from build123d import *

# Parameters (mm, degrees)
SKETCH1_W           = 85
SKETCH1_H           = 70
SKETCH1_R           = 1.375
SKETCH1_R_2         = 4.125
SKETCH1_R_3         = 3
SKETCH1_R_4         = 1.875
SKETCH1_R_5         = 2
BOSS_EXTRUDE4_DEPTH = 4
SKETCH1_7_R         = 4.5
CUT_EXTRUDE2_DEPTH  = 2


with BuildPart() as part:
    # Sketch1 → Boss-Extrude4 (new body)
    with BuildSketch(Plane(origin=(0, 0, 0), x_dir=(1, 0, 0), z_dir=(0, 1, 0))):
        Rectangle(SKETCH1_W, SKETCH1_H)
        with Locations((-27.5, 25)):
            Circle(SKETCH1_R, mode=Mode.SUBTRACT)
        with Locations((22.5, 25)):
            Circle(SKETCH1_R, mode=Mode.SUBTRACT)
        with Locations((22.5, -24.60667729)):
            Circle(SKETCH1_R, mode=Mode.SUBTRACT)
        with Locations((-27.5, -24.60667729)):
            Circle(SKETCH1_R, mode=Mode.SUBTRACT)
        with Locations((-15.52, 1)):
            Circle(SKETCH1_R_2, mode=Mode.SUBTRACT)
        with Locations((16.478339488, 0.999882702)):
            Circle(SKETCH1_R_3, mode=Mode.SUBTRACT)
        with Locations((9.407211052, 18.471043068)):
            Circle(SKETCH1_R_4, mode=Mode.SUBTRACT)
        with Locations((9.401398241, -16.528956449)):
            Circle(SKETCH1_R_5, mode=Mode.SUBTRACT)
    extrude(amount=BOSS_EXTRUDE4_DEPTH)

    # Sketch1_7 → Cut-Extrude2 (cut)
    with BuildSketch(Plane(origin=(0, 0, 0), x_dir=(1, 0, 0), z_dir=(0, 1, 0))):
        with Locations((16.478339488, 0.999882702)):
            Circle(SKETCH1_7_R)
    extrude(amount=CUT_EXTRUDE2_DEPTH, mode=Mode.SUBTRACT)


solid = part.part
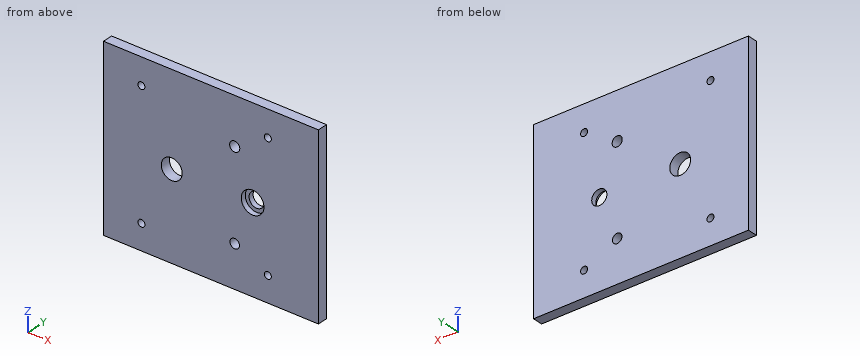
Input: part model. Units: mm. Frame: model coordinates. Coordinates: 2 decimals unless noted, no trailing zeros. Loops run counter-clockwise (first coordinate to the right, second up) from the corner with the lowest first, then second, coordinate; pieces in that order, holes last. Notation, with made-up numbers: (-13, 60) -> (40, 60) arc R6 cw to (40, 71) -> close; hole circle Ø9 at (-37, 80). An arc over 180 degrees is marked (long way). One line per item, written item: value.
(1) Pin query (flat end, axial travel): pin 1 Ø2.5 at (x, z) = (17.5, -3) entering from -Y. Return the tip coordinate at first contact, or that it passes through.
Answer below:
pin 1: stops at y = 2
(2) Ray query, line 1 along Z through (x, y) = (-27.5, 1.4) (3 decimals); line 2 along X through (y, z) = (2.05, -25) (3 decimals); line 3 along X through (y, z) = (1.2, -26). Return the intervals inside material, ascending.
Answer below:
line 1: z = -35 to -26.375, -23.625 to 23.232, 25.982 to 35
line 2: x = -42.5 to -28.875, -26.125 to 21.125, 23.875 to 42.5
line 3: x = -42.5 to -28.44, -26.56 to 21.56, 23.44 to 42.5
(3) Cut plane C-C (x = -15.52). Output: boundary loops of the cut face in (y, z) (3 decimals).
Answer below:
outline: (0, -35) -> (4, -35) -> (4, -5.125) -> (0, -5.125) -> close; (0, 3.125) -> (4, 3.125) -> (4, 35) -> (0, 35) -> close
(4) Cut plane B-B (z = -25). Output: boundary loops of the cut face in (x, y) (3 decimals).
Answer below:
outline: (-42.5, 0) -> (-28.875, 0) -> (-28.875, 4) -> (-42.5, 4) -> close; (-26.125, 0) -> (21.125, 0) -> (21.125, 4) -> (-26.125, 4) -> close; (23.875, 0) -> (42.5, 0) -> (42.5, 4) -> (23.875, 4) -> close
(5) Cut plane D-D (y = 2.6). Give the number of separate pieces and of enclosed holes in the cut face, then the cut area to 3 significant figures.
Answer below:
separate pieces: 1
enclosed holes: 8
area: 5,820 mm2
(6) Cut plane A-A (x = 22.5). Output: boundary loops of the cut face in (y, z) (3 decimals), then the cut area to 3 significant figures.
Answer below:
outline: (0, -35) -> (4, -35) -> (4, -26.375) -> (0, -26.375) -> close; (0, -23.625) -> (4, -23.625) -> (4, 23.232) -> (0, 23.232) -> close; (0, 25.982) -> (4, 25.982) -> (4, 35) -> (0, 35) -> close
area: 258 mm2
